from build123d import *

# Parameters (mm, degrees)
BASE_FLANGE1_DEPTH               = 160.02
SKETCH17_W                       = 196.85
SKETCH17_H                       = 12.7
BOSS_EXTRUDE2_DEPTH              = 3.175
EDGE_FLANGE1_STRIP_W             = 19.05
EDGE_FLANGE1_STRIP_H             = 3.175
EDGE_FLANGE1_STRIP_CUT_DEPTH     = 196.85
EDGE_FLANGE1_DEPTH               = 196.85
CUT_EXTRUDE3_REACH               = 291.036
SKETCH24_R                       = 2.5796875
SKETCH24_W                       = 45.72
SKETCH24_H                       = 50.8
SKETCH24_W_2                     = 38.1
SKETCH24_W_3                     = 25.4
F_13_64_0_20313_DIAMETER_HOLE1_D = 5.159502
CUT_EXTRUDE4_REACH               = 291.036
SKETCH28_W                       = 109.22
SKETCH28_H                       = 50.8
SKETCH29_W                       = 69.85
SKETCH29_H                       = 12.7
SKETCH29_W_2                     = 50.8
CUT_EXTRUDE5_DEPTH               = 290.035929254
CHAMFER1_SIZE                    = 12.7
CHAMFER1_SIZE2                   = 25.4


# Sheet-metal steps are written as plain solids
with BuildPart() as part:
    # Sketch7 → Base-Flange1 (new body)
    with BuildSketch(Plane.XY):
        with BuildLine():
            Line((-228.6, 38.1), (-228.6, 6.35))
            ThreePointArc((-228.6, 6.35), (-226.740128061, 1.859871939), (-222.25, 0))
            Line((-222.25, 0), (-6.35, 0))
            ThreePointArc((-6.35, 0), (-1.859871939, 1.859871939), (0, 6.35))
            Line((0, 6.35), (0, 38.1))
            Line((0, 38.1), (-3.175, 38.1))
            Line((-3.175, 38.1), (-3.175, 6.35))
            ThreePointArc((-3.175, 6.35), (-4.10493597, 4.10493597), (-6.35, 3.175))
            Line((-6.35, 3.175), (-222.25, 3.175))
            ThreePointArc((-222.25, 3.175), (-224.49506403, 4.10493597), (-225.425, 6.35))
            Line((-225.425, 6.35), (-225.425, 38.1))
            Line((-225.425, 38.1), (-228.6, 38.1))
        make_face()
    extrude(amount=BASE_FLANGE1_DEPTH)

    # Sketch17 → Boss-Extrude2 (add)
    with BuildSketch(Plane(origin=(0, 3.175, 0), x_dir=(1, 0, 0), z_dir=(0, 1, 0))):
        with Locations((-114.3, -166.37)):
            Rectangle(SKETCH17_W, SKETCH17_H)
    boss_extrude2 = extrude(amount=-BOSS_EXTRUDE2_DEPTH)

    # Edge-Flange1 strip (across the edge) → Edge-Flange1 strip cut (cut)
    with BuildSketch(Plane(origin=(-212.725, 3.175, 172.72), x_dir=(0, 0, -1), z_dir=(1, 0, 0))):
        with Locations((-3.175, -1.5875)):
            Rectangle(EDGE_FLANGE1_STRIP_W, EDGE_FLANGE1_STRIP_H)
    edge_flange1_strip_cut = extrude(amount=EDGE_FLANGE1_STRIP_CUT_DEPTH, mode=Mode.SUBTRACT)

    # Edge-Flange1 section (across the edge) → Edge-Flange1 (add)
    with BuildSketch(Plane(origin=(-212.725, 3.175, 172.72), x_dir=(0, 0, -1), z_dir=(1, 0, 0))):
        with BuildLine():
            Line((0, 3.175), (0, 17.145))
            Line((0, 17.145), (3.175, 17.145))
            Line((3.175, 17.145), (3.175, 3.175))
            ThreePointArc((3.175, 3.175), (4.10493597, 0.92993597), (6.35, 0))
            Line((6.35, 0), (6.35, -3.175))
            ThreePointArc((6.35, -3.175), (1.859871939, -1.315128061), (0, 3.175))
        make_face()
    edge_flange1 = extrude(amount=EDGE_FLANGE1_DEPTH)

    # Mirror1: Boss-Extrude2, Edge-Flange1 strip cut, Edge-Flange1 across plane
    add(boss_extrude2.mirror(Plane.XY.offset(80.01)))
    add(edge_flange1_strip_cut.mirror(Plane.XY.offset(80.01)), mode=Mode.SUBTRACT)
    add(edge_flange1.mirror(Plane.XY.offset(80.01)))

    # Cut-Extrude3: up to this face of the body (flat: up to its plane)
    cut_extrude3_end = Plane(part.part.faces().sort_by_distance((-212.725, 2.935376879, 163.195))[0])
    # Sketch24 → Cut-Extrude3 (cut, up to the picked face)
    with BuildSketch(Plane.ZY.offset(228.6), mode=Mode.PRIVATE) as cut_extrude3_sk1:
        with Locations(Location((33.02, 30.48, 0), (0, 0, 180))):
            Circle(SKETCH24_R)
    cut_extrude3_tool1 = split(extrude(cut_extrude3_sk1.sketch, amount=-CUT_EXTRUDE3_REACH, mode=Mode.PRIVATE), bisect_by=cut_extrude3_end, keep=Keep.BOTH, mode=Mode.PRIVATE)
    # Sketch24 → Cut-Extrude3 (cut, up to the picked face)
    with BuildSketch(Plane.ZY.offset(228.6), mode=Mode.PRIVATE) as cut_extrude3_sk2:
        with Locations(Location((114.3, 30.48, 0), (0, 0, 180))):
            Circle(SKETCH24_R)
    cut_extrude3_tool2 = split(extrude(cut_extrude3_sk2.sketch, amount=-CUT_EXTRUDE3_REACH, mode=Mode.PRIVATE), bisect_by=cut_extrude3_end, keep=Keep.BOTH, mode=Mode.PRIVATE)
    # Sketch24 → Cut-Extrude3 (cut, up to the picked face)
    with BuildSketch(Plane.ZY.offset(228.6), mode=Mode.PRIVATE) as cut_extrude3_sk3:
        with Locations((73.66, 12.7)):
            Rectangle(SKETCH24_W, SKETCH24_H)
    cut_extrude3_tool3 = split(extrude(cut_extrude3_sk3.sketch, amount=-CUT_EXTRUDE3_REACH, mode=Mode.PRIVATE), bisect_by=cut_extrude3_end, keep=Keep.BOTH, mode=Mode.PRIVATE)
    # Sketch24 → Cut-Extrude3 (cut, up to the picked face)
    with BuildSketch(Plane.ZY.offset(228.6), mode=Mode.PRIVATE) as cut_extrude3_sk4:
        with Locations((140.97, 12.7)):
            Rectangle(SKETCH24_W_2, SKETCH24_H)
    cut_extrude3_tool4 = split(extrude(cut_extrude3_sk4.sketch, amount=-CUT_EXTRUDE3_REACH, mode=Mode.PRIVATE), bisect_by=cut_extrude3_end, keep=Keep.BOTH, mode=Mode.PRIVATE)
    # Sketch24 → Cut-Extrude3 (cut, up to the picked face)
    with BuildSketch(Plane.ZY.offset(228.6), mode=Mode.PRIVATE) as cut_extrude3_sk5:
        with Locations((12.7, 12.7)):
            Rectangle(SKETCH24_W_3, SKETCH24_H)
    cut_extrude3_tool5 = split(extrude(cut_extrude3_sk5.sketch, amount=-CUT_EXTRUDE3_REACH, mode=Mode.PRIVATE), bisect_by=cut_extrude3_end, keep=Keep.BOTH, mode=Mode.PRIVATE)
    add(cut_extrude3_tool1.solids().sort_by(Axis((-228.6, 30.48, 33.02), (1, 0, 0)))[0], mode=Mode.SUBTRACT)
    add(cut_extrude3_tool2.solids().sort_by(Axis((-228.6, 30.48, 114.3), (1, 0, 0)))[0], mode=Mode.SUBTRACT)
    add(cut_extrude3_tool3.solids().sort_by(Axis((-228.6, 12.7, 73.66), (1, 0, 0)))[0], mode=Mode.SUBTRACT)
    add(cut_extrude3_tool4.solids().sort_by(Axis((-228.6, 12.7, 140.97), (1, 0, 0)))[0], mode=Mode.SUBTRACT)
    add(cut_extrude3_tool5.solids().sort_by(Axis((-228.6, 12.7, 12.7), (1, 0, 0)))[0], mode=Mode.SUBTRACT)

    # 13/64 (0.20313) Diameter Hole1 (through all)
    with Locations(Plane(origin=(0, 0, 0), x_dir=(0, 0, -1), z_dir=(1, 0, 0))):
        with Locations((-147.32, 30.48), (-12.7, 30.48)):
            Hole(F_13_64_0_20313_DIAMETER_HOLE1_D / 2)

    # Cut-Extrude4: up to this face of the body (flat: up to its plane)
    cut_extrude4_end = Plane(part.part.faces().sort_by_distance((-15.875, 2.935376879, -3.175))[0])
    # Sketch28 → Cut-Extrude4 (cut, up to the picked face)
    with BuildSketch(Plane(origin=(0, 0, 0), x_dir=(0, 0, -1), z_dir=(1, 0, 0)), mode=Mode.PRIVATE) as cut_extrude4_sk1:
        with Locations((-80.01, 12.7)):
            Rectangle(SKETCH28_W, SKETCH28_H)
    cut_extrude4_tool1 = split(extrude(cut_extrude4_sk1.sketch, amount=-CUT_EXTRUDE4_REACH, mode=Mode.PRIVATE), bisect_by=cut_extrude4_end, keep=Keep.BOTH, mode=Mode.PRIVATE)
    add(cut_extrude4_tool1.solids().sort_by(Axis((0, 12.7, 80.01), (-1, 0, 0)))[0], mode=Mode.SUBTRACT)

    # Sketch29 → Cut-Extrude5 (cut, through all)
    with BuildSketch(Plane(origin=(0, 0, 0), x_dir=(-1, 0, 0), z_dir=(0, -1, 0))):
        with Locations((88.9, -166.37)):
            Rectangle(SKETCH29_W, SKETCH29_H)
        with Locations((88.9, 6.35)):
            Rectangle(SKETCH29_W, SKETCH29_H)
        with Locations((187.325, -166.37)):
            Rectangle(SKETCH29_W_2, SKETCH29_H)
        with Locations((187.325, 6.35)):
            Rectangle(SKETCH29_W_2, SKETCH29_H)
    extrude(amount=-CUT_EXTRUDE5_DEPTH, mode=Mode.SUBTRACT)

    # Chamfer1
    chamfer1_edges = [part.edges().sort_by_distance(p)[0] for p in [
        (-227.0125, 38.1, 50.8),
    ]]
    chamfer1_side = [part.faces().sort_by_distance(p)[0] for p in [
        (-227.0125, 38.1, 38.1),
    ]]
    chamfer(chamfer1_edges, length=CHAMFER1_SIZE, length2=CHAMFER1_SIZE2, reference=chamfer1_side[0])


solid = part.part
Input: part model. Units: mm. Frame: model coordinates. A direction names the side the tool comes from. Give positions to 0.01 mm unless a question says otherwise; leave off trailing zeros. Write each loop counter-clockwise with the first axis right and the second up, starting at its lowest first coordinate (ties: lowest second). Pieces come first, ordered by that corner, then holes. Notation, with made-up numbers: (-22.75, -19) -> (2.25, -19) arc R11 ccw to (2.25, 0) -> close; hole circle Ø5 at (-38, 39.5). An arc over 180 degrees is marked (long way). Use one line per item in the form item = value. Start each with the question number.
1) Section query B-B on z = 12.7. Return the cut outline in (x, y) (3 decimals).
2) Section query C-C on x = -142. Return the cut outline in (y, z) (3 decimals), then the cut area to 3 significant figures.
3) Ray query, probe 1 along Z at (x, y) = (-1, 30); probe 2 along Z at (x, y) = (-129.5, 11) (3 decimals); probe 3 along Z at (x, y) = (-227, 30). Return the intervals inside material, ascending. Write a range as from..to.
4) Set-up query: faces 1 (the flat face through (-143, 13, -9.525)), 2 (the flat face through (-226, 15, 96.52)), 3 (the flat face through (-226, 15, 121.92)). Return all of +Z, -Z, +X, -X, +Y, -Y with unobstructed straight access to the full face (end or side cutting, diameter ignored); none if empty.
5) Pin query (flat end, axial travel): pin 1 (4 mm diameter, centred on y = 30.48, z = 114.3, fed in from +X); pin 2 (1 mm diameter, centred on x = -38.5, z = -12, fed in from +Y); pin 3 (1 mm diameter, centred on y = 2.5, z = 132.5, fed in from -X) (3 decimals); pin 4 (1.6 mm diameter, centred on x = -175.5, y = 2.5, fed in from -Z). Return the tip coordinate at first contact, or that it passes through.
6) Draft query along Y for faces 4 (the flat face through (-227.03, 25.22, 44.54)), 5 (the cylindrical face through (-143.14, 1.81, -10.79)), 6 (the cylindrical face through (-1.61, 32.655, 14.087)), 7 (the flat face through (-143, 13, 169.545)). Return one class per face: pulls with the +Y half, pulls with the -Y half, needs draft (parallel to the pull), parting line crosses it, or undercut.
7) Section query D-D on z = 114.3. Return the cut outline in (x, y) (3 decimals), then the cut area to 3 significant figures.
8) Section query A-A on y = 30.48. Count the separate pieces of the cut face and the enclosed holes in it, then the cut area to 3 significant figures.
Outcome:
q1.outline = (-212.725, 0) -> (-6.35, 0) arc R6.35 ccw to (0, 6.35) -> (0, 27.9) -> (-3.175, 27.9) -> (-3.175, 6.35) arc R3.175 cw to (-6.35, 3.175) -> (-212.725, 3.175) -> close; (-3.175, 33.06) -> (0, 33.06) -> (0, 38.1) -> (-3.175, 38.1) -> close
q2.outline = (0, -6.35) arc R6.35 ccw to (6.35, -12.7) -> (20.32, -12.7) -> (20.32, -9.525) -> (6.35, -9.525) arc R3.175 cw to (3.175, -6.35) -> (3.175, 166.37) arc R3.175 cw to (6.35, 169.545) -> (20.32, 169.545) -> (20.32, 172.72) -> (6.35, 172.72) arc R6.35 ccw to (0, 166.37) -> close
q2.area = 685 mm^2
q3.probe_1 = 0..10.17, 15.23..25.4, 134.62..144.79, 149.85..160.02
q3.probe_2 = -12.7..-9.525, 169.545..172.72
q3.probe_3 = 25.4..30.49, 35.55..42.15, 96.52..111.77, 116.83..121.92
q4.face_1 = +X, -X, +Y
q4.face_2 = -X, +Y, -Y
q4.face_3 = +Z, -X, +Y, -Y
q5.pin_1 = through
q5.pin_2 = 20.32
q5.pin_3 = -212.725
q5.pin_4 = 0
q6.face_4 = pulls with the +Y half
q6.face_5 = pulls with the -Y half
q6.face_6 = undercut
q6.face_7 = needs draft
q7.outline = (-228.6, 6.35) arc R6.35 ccw to (-222.25, 0) -> (-15.875, 0) -> (-15.875, 3.175) -> (-222.25, 3.175) arc R3.175 cw to (-225.425, 6.35) -> (-225.425, 27.9) -> (-228.6, 27.9) -> close; (-228.6, 33.06) -> (-225.425, 33.06) -> (-225.425, 38.1) -> (-228.6, 38.1) -> close
q7.area = 763 mm^2
q8.separate_pieces = 8
q8.enclosed_holes = 0
q8.area = 229 mm^2
